Here's the drawing with two shaded views (mm, measured from the low corner). I have some questions. A direction names the side the tool comes from. Coordinates: 2 decimals unless noted, no trailing zeros. Write each loop counter-clockwise with the first axis right and the second up, starting at its lowest first coordinate (ties: lowest second). Pieces come first, ordered by that corner, then holes.
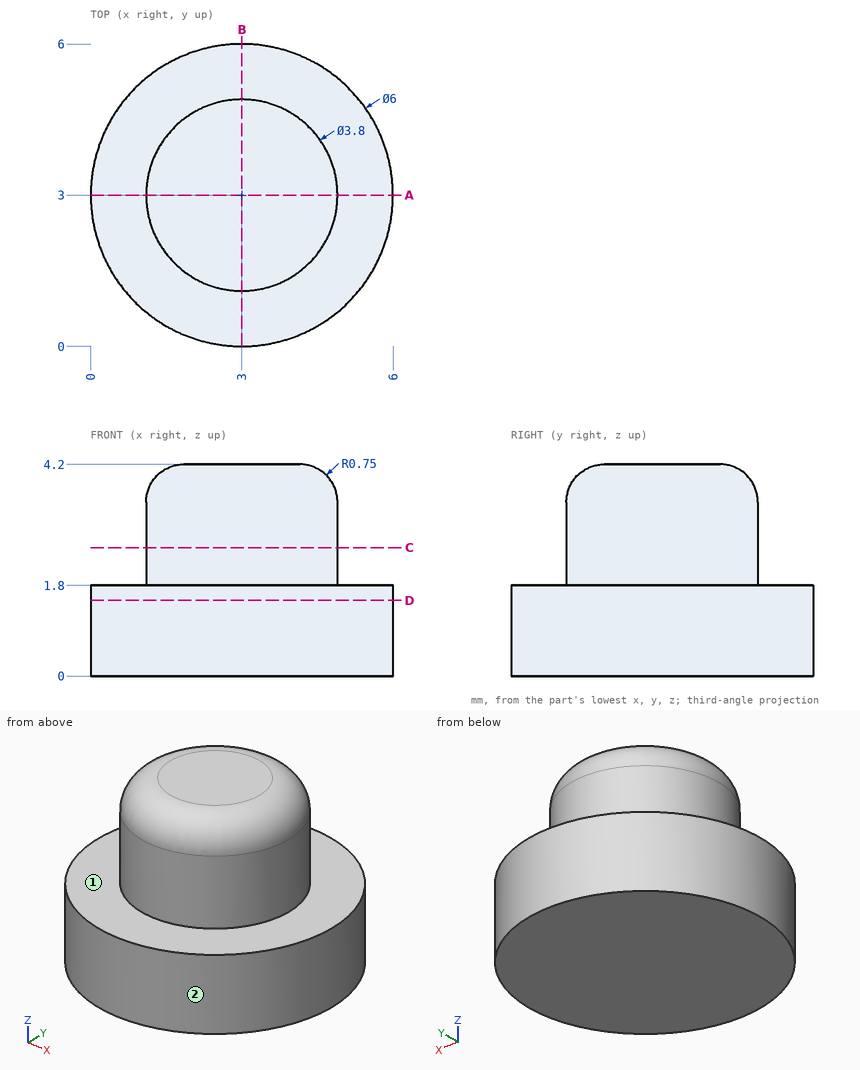
1. If we section it at C-C, the plane z = 2.55: List the corners of the cut face in (x, y) for me.
2. If we section it at A-A, the plane y = 3: List the corners of the cut face in (x, z) for me, plus the area to 3 significant figures.
3. If I drill on L1, parallel to Z at x = 2, y = 4.95; L2, parallel to Y at x = 2.9, z = 1.25; L3, parallel to X at y = 2.9, z = 2.95, over which ranges is the centre line in solid material (lowest first)?
4. If we section it at D-D, the plane z = 1.5: List the corners of the cut face in (x, y) for me, plus the area to 3 significant figures.
5. Which directions (+Z, -Z, +X, -X, +Y, -Y) give clear straight access to the entire face, cutting with the end or side of a thin tool? Please do the marked faces 1 and 2.
6. I'm going to push flat-ended pins straight in: P1, Ø2, axis at x = 5, z = 2.5, coming from the -Y side; P2, Ø1.5, axis at x = 3, z = 2.5, coming from the -Y side; P3, Ø1, axis at x = 2, y = 1, coming from the +Z side; P4, Ø2, axis at y = 4.5, z = 2, coming from the +X side. Where does each tip first touch, or does it pass through?
Answers:
1. outline: circle Ø3.8 at (3, 3)
2. outline: (0, 0) - (6, 0) - (6, 1.8) - (4.9, 1.8) - (4.9, 3.45) arc R0.75 ccw to (4.15, 4.2) - (1.85, 4.2) arc R0.75 ccw to (1.1, 3.45) - (1.1, 1.8) - (0, 1.8) - close
2. area: 19.7 mm2
3. L1: z = 0 to 1.8
3. L2: y = 0 to 6
3. L3: x = 1.1 to 4.9
4. outline: circle Ø6 at (3, 3)
4. area: 28.3 mm2
5. face 1: +Z
5. face 2: +Z, -Z
6. P1: stops at y = 0.29
6. P2: stops at y = 0
6. P3: stops at z = 3.92
6. P4: stops at x = 5.95
